Geometry: final body of the model. Coordinates: model frame, mm. Give positions to 0.01 mm unless a question says otherwise; leave off trailing zeros. Order: outer loops, then holes, each group sorted by start corner. A loop starts at its lowest first (then second) coordinate and runs counter-clockwise, first axis right, second up. Notation, with made-up numbers: (-22.75, 80) -> (15.25, 80) arc R8 ccw to (15.25, 84) -> close; hole circle Ø4 at (62, 65.25). An arc over 180 degrees is marked (long way). Answer in a Markdown table with one row per item. Add a question column.
Q1. Cut plane B-B on x = 5. Return the cut outline in (y, z).
Q2. Line query: line 1 along Z through (x, y) = (5, -8.5); line 2 along X through (y, z) = (-7.7, -345); line 3 along Z through (x, y) = (4.5, -4.5). Output: solid intervals per line, ascending. Write a range as from..to.
Q3. Cut plane A-A on y = -2.5. Return the cut outline in (x, z), and give its area (3 significant figures).
Q4. Contact query for flat-ended pins moving along their axis: P1, Ø5, axis at x = 6, z = -3.5, coming from the +Y side; P2, Ø1.2, axis at x = 5, z = 344, coming from the +Y side; P3, Ø2.5, axis at x = 4.5, y = -3.5, coming from the -Z side. Output: stop coordinate, or through.
from build123d import *

# Parameters (mm, degrees)
F1_DEPTH = 10
F2_R     = 2
F3_DEPTH = 4.5
F5_W     = 5
F5_H     = 10
F6_DEPTH = 10.001
F7_R     = 2
F8_DEPTH = 4.5


with BuildPart() as f1:
    # F0 (on Right) → F1 (new body)
    with BuildSketch(Plane.YZ):
        Polygon((-10, 0), (0, 0), (0, 340), (-5, 340), (-5, 350), (-10, 350), align=None)
    extrude(amount=F1_DEPTH)

    # F2 (on face) → F3 (cut)
    with BuildSketch(Plane(origin=(0, -5, 0), x_dir=(-1, 0, 0), z_dir=(0, 1, 0))):
        with Locations((-5, 345)):
            Circle(F2_R)
    extrude(amount=-F3_DEPTH, mode=Mode.SUBTRACT)

    # F4: F1 across plane


with BuildPart() as f1_1:
    add(f1.part)
    add(f1.part.mirror(Plane.XY))

    # F5 (on face) → F6 (cut, through all)
    with BuildSketch(Plane.YZ.offset(10)):
        with Locations((-2.5, -5)):
            Rectangle(F5_W, F5_H)
    extrude(amount=-F6_DEPTH, mode=Mode.SUBTRACT)

    # F7 (on face) → F8 (cut)
    with BuildSketch(Plane(origin=(0, -5, 0), x_dir=(-1, 0, 0), z_dir=(0, 1, 0))):
        with Locations((-5, -5)):
            Circle(F7_R)
    extrude(amount=-F8_DEPTH, mode=Mode.SUBTRACT)


solid = f1_1.part
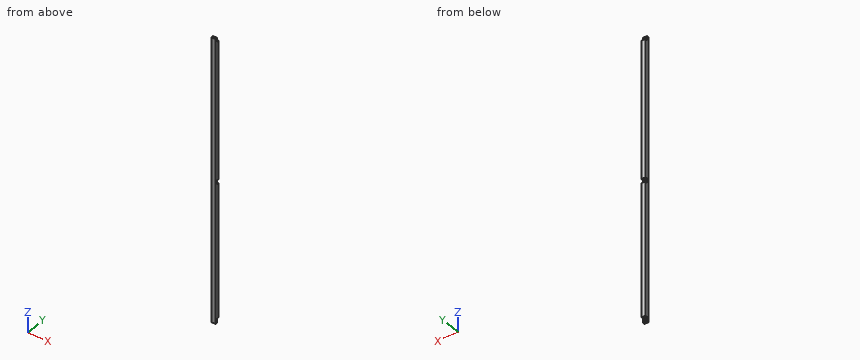
Completed:
| question | item | result |
|---|---|---|
| 1 | outline | (-10, -350) -> (-5, -350) -> (-5, -347) -> (-9.5, -347) -> (-9.5, -343) -> (-5, -343) -> (-5, -340) -> (0, -340) -> (0, -10) -> (-5, -10) -> (-5, -7) -> (-9.5, -7) -> (-9.5, -3) -> (-5, -3) -> (-5, 0) -> (0, 0) -> (0, 340) -> (-5, 340) -> (-5, 343) -> (-9.5, 343) -> (-9.5, 347) -> (-5, 347) -> (-5, 350) -> (-10, 350) -> close |
| 2 | line 1 | z = -350..-347, -343..-7, -3..343, 347..350 |
| 2 | line 2 | x = 0..3, 7..10 |
| 2 | line 3 | z = -340..-10, 0..340 |
| 3 | outline | (0, -340) -> (10, -340) -> (10, -10) -> (0, -10) -> close; (0, 0) -> (10, 0) -> (10, 340) -> (0, 340) -> close |
| 3 | area | 6,700 mm² |
| 4 | P1 | stops at y = -5 |
| 4 | P2 | stops at y = -9.5 |
| 4 | P3 | stops at z = -340 |
